from build123d import *

# Parameters (mm, degrees)
F0_R     = 20
F0_R_2   = 15.75
F0_R_3   = 4
F1_DEPTH = 1
F2_DEPTH = 10


# Not quite as in the source:
# - a feature names something its author has since deleted; it is built from what else it names


with BuildPart() as f1:
    # F0 (on Front) → F1 (new body)
    with BuildSketch(Plane.XZ):
        Circle(F0_R)
        Circle(F0_R_2, mode=Mode.SUBTRACT)
        Circle(F0_R_2)
        Circle(F0_R_3, mode=Mode.SUBTRACT)
    extrude(amount=F1_DEPTH)

    # F0 (on Front) → F2 (join)
    with BuildSketch(Plane.XZ):
        Circle(F0_R_2)
        Circle(F0_R_3, mode=Mode.SUBTRACT)
    extrude(amount=-F2_DEPTH)


solid = f1.part
Check sheet for the modelled part. Datum: model origin and axes. Units: mm. A direction names the side the tool comes from. Give positions to 0.01 mm unless a question says otherwise; leave off trailing zeros. Order: outer loops, then holes, each group sorted by start corner. A loop starts at its lowest first (then second) coordinate and runs counter-clockwise, first axis right, second up. Notation, with made-up numbers: (32, -20) - (55, -20) arc R22 ccw to (55, 9) - close; hole circle Ø2 at (42, -33). An arc over 180 degrees is marked (long way). Answer as CSV lines item,"result".
1. Section check C-C (y = 2.25). Record the boundary of the cut face in (x, z).
Result sheet:
outline,"circle Ø31.5 at (0, 0); hole circle Ø8 at (0, 0)"
2. Tool access check on faces 1 (the face through (6, 0, -15)), 2 (the face through (3, 10, -3)). Record the directions out of +Z, -Z, +X, -X, +Y, -Y that give a thin tool (end or side, any length) a straight path to the whole face; none if there is none.
Result sheet:
face 1,"+Y"
face 2,"+Z, -Z, +X, -X, +Y"
3. Section check D-D (x = 8). Record the boundary of the cut face in (y, z).
Result sheet:
outline,"(-1, -18.33) - (0, -18.33) - (0, -13.57) - (10, -13.57) - (10, 13.57) - (0, 13.57) - (0, 18.33) - (-1, 18.33) - close"
4. Go/stop test with flat-tipped pins: P1, Ø3, axis at y = 7, z = -13.5, coming from the +X side; P2, Ø1.5, axis at y = 8, z = 4.5, coming from the +X side; P3, Ø2, axis at x = -2, y = 2, coming from the +Z side. Record where each tip stops, or that it passes through.
Result sheet:
P1,"x = 10.2"
P2,"x = 15.3"
P3,"z = 15.72"
5. Scan lines: probe 1 along Z at (x, y) = (0, 7.25); probe 2 along Z at (x, y) = (0, -0.35); probe 3 along Y at (x, z) = (13, -14). Record each from-to range of solid material in increasing order. Write a range as from..to.
Result sheet:
probe 1,"-15.75..-4, 4..15.75"
probe 2,"-20..-4, 4..20"
probe 3,"-1..0"
6. Section check A-A (z = 0). Record the boundary of the cut face in (x, y), then the cut area to 3 significant figures.
Result sheet:
outline,"(-20, -1) - (-4, -1) - (-4, 10) - (-15.75, 10) - (-15.75, 0) - (-20, 0) - close; (4, -1) - (20, -1) - (20, 0) - (15.75, 0) - (15.75, 10) - (4, 10) - close"
area,"267 mm²"
7. Section check B-B (x = 0). Record the boundary of the cut face in (y, z), then the cut area to 3 significant figures.
Result sheet:
outline,"(-1, -20) - (0, -20) - (0, -15.75) - (10, -15.75) - (10, -4) - (-1, -4) - close; (-1, 4) - (10, 4) - (10, 15.75) - (0, 15.75) - (0, 20) - (-1, 20) - close"
area,"267 mm²"
